```python
from build123d import *

# Parameters (mm, degrees)
SKETCH_W     = 75
SKETCH_H     = 31.75
PAD_DEPTH    = 4
SKETCH001_R  = 7.5
POCKET_DEPTH = 4.001
PAD001_DEPTH = 4


with BuildPart() as part:
    # Sketch → Pad (new body)
    with BuildSketch(Plane.XY):
        Rectangle(SKETCH_W, SKETCH_H)
    extrude(amount=PAD_DEPTH)

    # Sketch001 → Pocket (cut, through all)
    with BuildSketch(Plane.XY.offset(4)):
        with Locations((21.5, 0)):
            Circle(SKETCH001_R)
    extrude(amount=-POCKET_DEPTH, mode=Mode.SUBTRACT)

    # Sketch002 → Pad001 (new body)
    with BuildSketch(Plane.XY.offset(4)):
        Polygon((24.486536, 11.966792), (10.3444, -2.175344), (10.3444, 11.966792), align=None)
        Polygon((29.815649, 0.664607), (21.707865, 8.772391), (34.469826, 11.738337), align=None)
        Polygon((30.957856, 0.4776), (22.4028, -8.077456), (35.779438, -11.627933), align=None)
        Polygon((13.253763, -0.734019), (21.279048, -8.759304), (7.24554, -12.506914), align=None)
    extrude(amount=-PAD001_DEPTH)


solid = part.part
```
Geometry check sheet. Reference: the model listing, model coordinates, mm. A direction names the side the tool comes from. Coordinates: 2 decimals unless noted, no trailing zeros. Order: outer loops, then holes, each group sorted by start corner. A loop starts at its lowest first (then second) coordinate and runs counter-clockwise, first axis right, second up. Notation, with made-up numbers: M 47.25,35 L 104.25,35 A26 ccw 104.25,51 Z; hole C 17,-17.75 d1. An arc over 180 degrees is marked long. Answer as a JSON object with one key per item and string values.
Q1. Cross-section at C-C on x = 15.5. Record the cut outline in (y, z) (3 decimals), and give its area (3 significant figures).
Results are:
{"outline": "M -15.875,0 L -2.98,0 L -2.98,4 L -15.875,4 Z; M 2.98,0 L 15.875,0 L 15.875,4 L 2.98,4 Z", "area": "103 mm²"}
Q2. Cross-section at B-B on z = 2.1. Record the cut outline in (x, y) (3 decimals), and give its area (3 significant figures).
Results are:
{"outline": "M -37.5,-15.875 L 37.5,-15.875 L 37.5,15.875 L -37.5,15.875 Z; hole M 14.188,-1.668 L 19.832,-7.312 A7.5 ccw 23.168,-7.312 L 28.812,-1.668 A7.5 ccw 28.812,1.668 L 23.168,7.312 A7.5 ccw 19.832,7.312 L 14.188,1.668 A7.5 ccw Z", "area": "2,230 mm²"}
Q3. Cross-section at A-A on y = 0. Record the cut outline in (x, z), and give its area (3 significant figures).
Results are:
{"outline": "M -37.5,0 L 14,0 L 14,4 L -37.5,4 Z; M 29,0 L 37.5,0 L 37.5,4 L 29,4 Z", "area": "240 mm²"}
Q4. Release check for a two-part mould opening along X. For faces 3 (the flat face through (-37.5, 0, 2)), 4 (the flat face through (37.5, 0, 2)), 5 (the flat face through (16.97, -4.45, 2.03)), 6 (the flat face through (-1, 0, 0)) record: released by +X, released by -X, zero draft, split by the parting line, or undercut.
Results are:
{"face 3": "released by -X", "face 4": "released by +X", "face 5": "undercut", "face 6": "zero draft"}
Q5. Scan lines: line 1 (Y direction, x = 28, z = 3.15) (3 decimals); line 2 (X direction, y = 5.5, z = 3.8); line 3 (X direction, y = -4, z = 0.45). Record each from-to range of solid material in increasing order.
Results are:
{"line 1": "y = -15.875 to -2.48, 2.48 to 15.875", "line 2": "x = -37.5 to 18.02, 24.98 to 37.5", "line 3": "x = -37.5 to 16.52, 26.48 to 37.5"}
Q6. Tool access check on faces 1 (the flat face through (26.03, 4.45, 2.03)), 2 (the flat face through (1, 0, 4)). Record the directions out of +Z, -Z, +X, -X, +Y, -Y that give a thin tool (end or side, any length) a straight path to the whole face; none if there is none.
Results are:
{"face 1": "+Z, -Z", "face 2": "+Z, +X, -X, +Y, -Y"}
